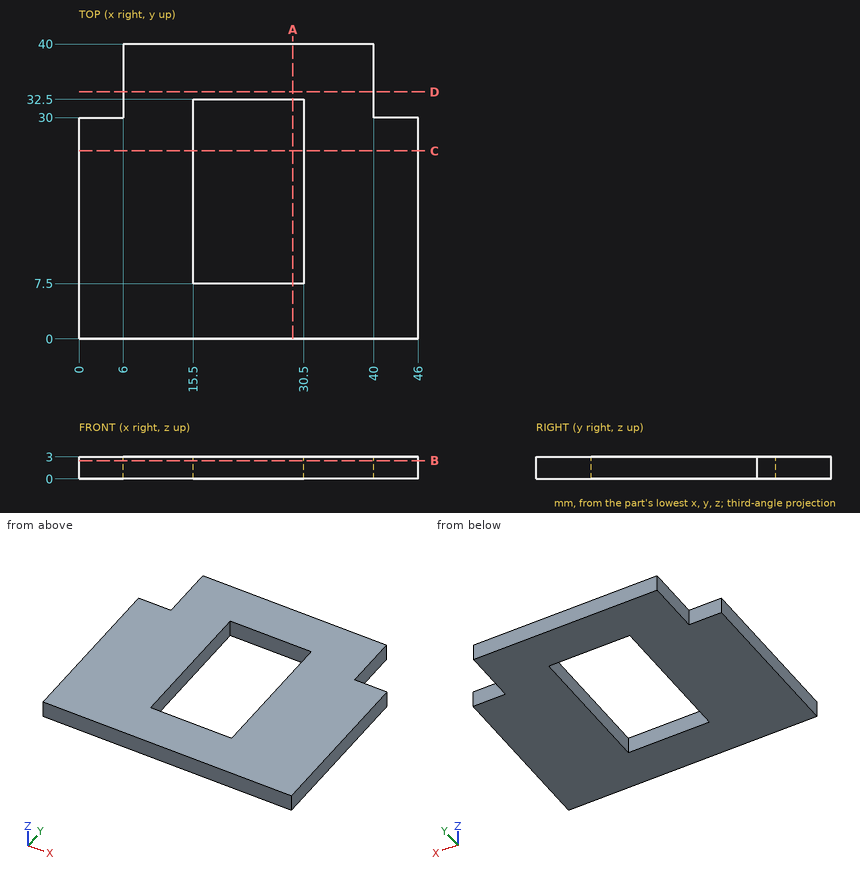
Can you work these out from the drawing? Everything is in mm from the part's minimum corner. Round coordinates to 2 decimals unless told otherwise and drop trailing zeros. Loops run counter-clockwise (first coordinate to the right, second up) from the corner with the lowest first, then second, coordinate; pieces in that order, holes last. Notation, with made-up numbers: M 86.25,87 L 99.25,87 A9 cw 99.25,96 Z; hole C 67,-27 d5. An arc over 180 degrees is marked long. Write item = value, one per line.
1. I want a section at B-B, the plane z = 2.5. Write out the boundary of the cut face in (x, y), and give its area (4 significant figures).
Results below:
outline = M 0,0 L 46,0 L 46,30 L 40,30 L 40,40 L 6,40 L 6,30 L 0,30 Z; hole M 15.5,7.5 L 30.5,7.5 L 30.5,32.5 L 15.5,32.5 Z
area = 1,345 mm²
2. I need wall thicknesses on probe 1 along X at (y, z) = (22.5, 2.55); probe 2 along Y at (x, z) = (26, 2.45); probe 3 along X at (y, z) = (35.5, 0.6). Which ranges of each line are inside material? Lowest first, please.
Results below:
probe_1 = 0 to 15.5, 30.5 to 46
probe_2 = 0 to 7.5, 32.5 to 40
probe_3 = 6 to 40
3. I want a section at C-C, the plane y = 25.5. Write out the boundary of the cut face in (x, z), and give its area (3 significant figures).
Results below:
outline = M 0,0 L 15.5,0 L 15.5,3 L 0,3 Z; M 30.5,0 L 46,0 L 46,3 L 30.5,3 Z
area = 93.0 mm²
4. I want a section at A-A, the plane x = 29. Write out the boundary of the cut face in (y, z), and give its area (3 significant figures).
Results below:
outline = M 0,0 L 7.5,0 L 7.5,3 L 0,3 Z; M 32.5,0 L 40,0 L 40,3 L 32.5,3 Z
area = 45.0 mm²
5. I want a section at D-D, the plane y = 33.5. Write out the boundary of the cut face in (x, z), and give its area (3 significant figures).
Results below:
outline = M 6,0 L 40,0 L 40,3 L 6,3 Z
area = 102 mm²
6. Will these pins go through, and if not, where does the flat tip stop? P1, Ø3, axis at x = 14.5, y = 15.5, coming from the -Z side; P2, Ø0.9, axis at x = 44.5, z = 1.5, coming from the +Y side.
Results below:
P1 = 0
P2 = 30
